Can you work these out from the drawing? Everything is in mm from the part's minimum corner. Give positions to 0.01 mm unless a question says otherwise; leave off trailing zeros. Write each loop counter-clockwise with the first axis right and the second up, starting at its lowest first coordinate (ties: lowest second). Pieces come first, ordered by that corner, then holes. Notation, with made-up numbers: (47.25, 28.5) - (61.25, 28.5) arc R18 ccw to (61.25, 43.5) - close; hole circle Ø1 at (46.5, 54.5). An arc over 180 degrees is marked (long way). Answer in a Markdown table with one row per item.
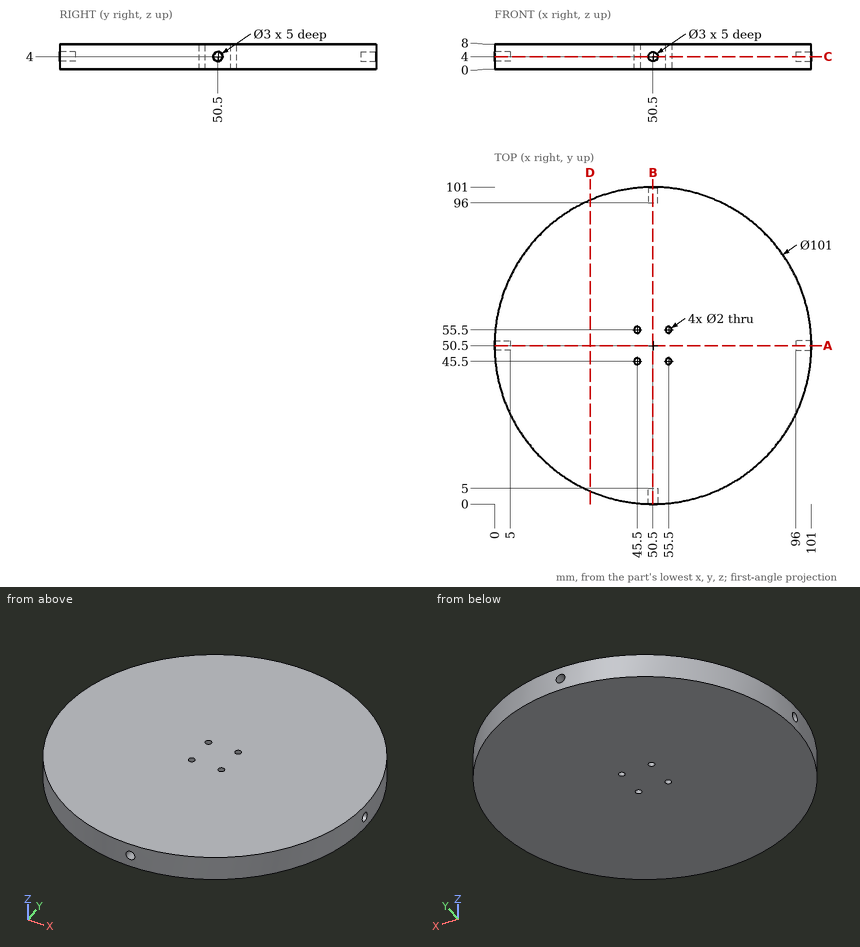
1) Imagine slicing it at C-C (z = 4). List the corners of the cut face in (x, y) for me.
Check values:
| item | result |
|---|---|
| outline | (0.02, 49) arc R50.5 ccw to (49, 0.02) - (49, 5) - (52, 5) - (52, 0.02) arc R50.5 ccw to (100.98, 49) - (96, 49) - (96, 52) - (100.98, 52) arc R50.5 ccw to (52, 100.98) - (52, 96) - (49, 96) - (49, 100.98) arc R50.5 ccw to (0.02, 52) - (5, 52) - (5, 49) - close; hole circle Ø2 at (45.5, 45.5); hole circle Ø2 at (45.5, 55.5); hole circle Ø2 at (55.5, 45.5); hole circle Ø2 at (55.5, 55.5) |
2) Will these pins go through, and if not, where does the flat tip stop? P1, Ø2, axis at y = 23.5, z = 3.5, coming from the +X side; P2, Ø2.5, axis at x = 55.5, y = 55.5, coming from the -Z side; P3, Ø1, axis at x = 21.5, z = 5.5, coming from the -Y side; P4, Ø2.5, axis at x = 50.5, z = 4, coming from the -Y side.
Check values:
| item | result |
|---|---|
| P1 | stops at x = 93.79 |
| P2 | stops at z = 0 |
| P3 | stops at y = 8.81 |
| P4 | stops at y = 5 |
3) Imagine slicing it at A-A (y = 50.5). List the corners of the cut face in (x, z) for me.
Check values:
| item | result |
|---|---|
| outline | (0, 0) - (101, 0) - (101, 2.5) - (96, 2.5) - (96, 5.5) - (101, 5.5) - (101, 8) - (0, 8) - (0, 5.5) - (5, 5.5) - (5, 2.5) - (0, 2.5) - close |
4) Imagine slicing it at D-D (x = 30.5). List the corners of the cut face in (y, z) for me.
Check values:
| item | result |
|---|---|
| outline | (4.13, 0) - (96.87, 0) - (96.87, 8) - (4.13, 8) - close |
5) If I drill on line 1 (Y direction, x = 45.5, z = 3.25); line 2 (Y direction, x = 5, z = 2.5); line 3 (Y direction, x = 15, z = 6), over which ranges is the centre line in solid material (lowest first)?
Check values:
| item | result |
|---|---|
| line 1 | y = 0.25 to 44.5, 46.5 to 54.5, 56.5 to 100.75 |
| line 2 | y = 28.59 to 72.41 |
| line 3 | y = 14.58 to 86.42 |
